from build123d import *

# Parameters (mm, degrees)
SKETCH_1_R          = 18
SKETCH_1_R_2        = 1.55
EXTRUDE_1_DEPTH     = 4
SKETCH_3_R          = 2.6
CUT_EXTRUDE_2_DEPTH = 2
CUT_EXTRUDE_3_DEPTH = 26.53429067
SKETCH_5_R          = 5.1
EXTRUDE_2_DEPTH     = 6
CUT_EXTRUDE_START   = 2.4
SKETCH_2_R          = 1.55
CUT_EXTRUDE_4_DEPTH = 2.4


with BuildPart() as part:
    # Sketch 1 → Extrude 1 (new body)
    with BuildSketch(Plane(origin=(0, 0, 0), x_dir=(1, 0, 0), z_dir=(0, 1, 0))):
        with Locations(Location((0, 0, 0), (0, 0, 270))):
            Circle(SKETCH_1_R)
        with Locations(Location((-12.124355653, -7, 0), (0, 0, 270))):
            Circle(SKETCH_1_R_2, mode=Mode.SUBTRACT)
        with Locations(Location((0, 14, 0), (0, 0, 270))):
            Circle(SKETCH_1_R_2, mode=Mode.SUBTRACT)
        with Locations(Location((12.124355653, -7, 0), (0, 0, 270))):
            Circle(SKETCH_1_R_2, mode=Mode.SUBTRACT)
    extrude(amount=EXTRUDE_1_DEPTH)

    # Sketch 3 → Cut-Extrude 2 (cut)
    with BuildSketch(Plane.XZ):
        with Locations(Location((0, 0, 0), (0, 0, 270))):
            Circle(SKETCH_3_R)
    extrude(amount=-CUT_EXTRUDE_2_DEPTH, mode=Mode.SUBTRACT)

    # Sketch 4 → Cut-Extrude 3 (cut, through all)
    with BuildSketch(Plane.XZ.offset(-2)):
        with BuildLine():
            ThreePointArc((2.6, 0), (-1.177768117, 2.317943542), (-1.532970972, -2.1))
            Line((-1.532970972, -2.1), (1.532970972, -2.1))
            ThreePointArc((1.532970972, -2.1), (2.317943542, -1.177768117), (2.6, 0))
        make_face()
    extrude(amount=-CUT_EXTRUDE_3_DEPTH, mode=Mode.SUBTRACT)

    # Sketch 5 → Extrude 2 (add)
    with BuildSketch(Plane(origin=(0, 4, 0), x_dir=(1, 0, 0), z_dir=(0, 1, 0))):
        with Locations(Location((0, 0, 0), (0, 0, 270))):
            Circle(SKETCH_5_R)
        with BuildLine():
            Line((-1.532970972, 2.1), (1.532970972, 2.1))
            ThreePointArc((1.532970972, 2.1), (0, -2.6), (-1.532970972, 2.1))
        make_face(mode=Mode.SUBTRACT)
    extrude(amount=EXTRUDE_2_DEPTH)

    # Sketch 2 → Cut-Extrude 4 (cut)
    # profile 1 of 3: a face of its own
    with BuildSketch(Plane.XZ.offset(-4).offset(CUT_EXTRUDE_START)):
        Polygon((-8.891194146, 7), (-10.507774899, 9.8), (-13.740936407, 9.8), (-15.35751716, 7), (-13.740936407, 4.2), (-10.507774899, 4.2), align=None)
        with Locations(Location((-12.124355653, 7, 0), (0, 0, 270))):
            Circle(SKETCH_2_R, mode=Mode.SUBTRACT)
    # profile 2 of 3: a face of its own
    with BuildSketch(Plane.XZ.offset(-4).offset(CUT_EXTRUDE_START)):
        Polygon((-1.616580754, -11.2), (-3.233161507, -14), (-1.616580754, -16.8), (1.616580754, -16.8), (3.233161507, -14), (1.616580754, -11.2), align=None)
        with Locations(Location((0, -14, 0), (0, 0, 270))):
            Circle(SKETCH_2_R, mode=Mode.SUBTRACT)
    # profile 3 of 3: a face of its own
    with BuildSketch(Plane.XZ.offset(-4).offset(CUT_EXTRUDE_START)):
        Polygon((10.507774899, 4.2), (13.740936407, 4.2), (15.35751716, 7), (13.740936407, 9.8), (10.507774899, 9.8), (8.891194146, 7), align=None)
        with Locations(Location((12.124355653, 7, 0), (0, 0, 270))):
            Circle(SKETCH_2_R, mode=Mode.SUBTRACT)
    extrude(amount=-CUT_EXTRUDE_4_DEPTH, mode=Mode.SUBTRACT)


solid = part.part
CAD build for the part. Positions are in the model's coordinates, mm. A direction names the side the tool comes from. Give positions to 0.01 mm unless a question says otherwise; leave off trailing zeros. Write each loop counter-clockwise with the first axis right and the second up, starting at its lowest first coordinate (ties: lowest second). Pieces come first, ordered by that corner, then holes. Notation, with made-up numbers: M -21,42.5 L 14,42.5 A22 ccw 14,62.5 Z; hole C 14.25,57 d6. An arc over 180 degrees is marked long. Put each result on its own line as item: value. Start each with the question number.
(1) Band-saw the part on A-A, the plane x = 0. Write the cut outline in (y, z), and give its area (3 significant figures).
(2) Band-saw the part on D-D, the plane z = 9. Write the cut outline in (x, y).
(3) Flat gauge pins, fed straight in: pin 1 Ø4 at (x, z) = (0, 0) entering from -Y; pin 2 Ø3 at (x, z) = (-0.5, -13) entering from +Y; pin 3 Ø1.9 at (x, y) = (-12.5, 3) entering from -Z; pin 4 Ø6 at (x, z) = (-7, -13) entering from +Y. Where does each tip first touch, or does it go through?
(4) Band-saw the part on C-C, the plane x = 11. Write the cut outline in (y, z).
(5) Band-saw the part on B-B, the plane y = 3.5. Write the cut outline in (x, z), and give its area (3 significant figures).
(6) Probe L1, parallel to Z at x = 1, y = 3.5; L2, parallel to X at y = 3.5, z = 0; L3, parallel to X at y = 1.2, z = 7. List the from-to ranges inside material, lowest first.
(7) Mould opens along X. For faces 4 (the face through (-14.538, 2.783, 8.42)), 5 (the face through (14.538, 2.783, 5.58)), 6 (the face through (-4, 4, 4)) say: +X half, -X half, draft (parallel to the pull), parting line (faces both ways), or undercut.
(8) Which spindle directions (+Z, -Z, +X, -X, +Y, -Y) get a long thin tool onto all of the face, cutting with end or side? Do faces 1 (the face through (0, 6, -2.1)), 2 (the face through (-12, 3, 4.2)), 3 (the face through (-4, 0, 0)). Say none if no direction does.
Response values:
1. outline: M 0,-18 L 4,-18 L 4,-16.8 L 1.6,-16.8 L 1.6,-15.55 L 0,-15.55 Z; M 0,-12.45 L 1.6,-12.45 L 1.6,-11.2 L 4,-11.2 L 4,-5.1 L 10,-5.1 L 10,-2.1 L 2,-2.1 L 2,-2.6 L 0,-2.6 Z; M 0,2.6 L 10,2.6 L 10,5.1 L 4,5.1 L 4,18 L 0,18 Z
1. area: 139 mm2
2. outline: M -15.59,0 L 15.59,0 L 15.59,4 L 14.2,4 L 14.2,1.6 L 10.05,1.6 L 10.05,4 L -10.05,4 L -10.05,1.6 L -14.2,1.6 L -14.2,4 L -15.59,4 Z
3. pin 1: passes through
3. pin 2: stops at y = 1.6
3. pin 3: stops at z = -13.81
3. pin 4: stops at y = 4
4. outline: M 0,-14.25 L 4,-14.25 L 4,4.2 L 1.6,4.2 L 1.6,5.93 L 0,5.93 Z; M 0,8.07 L 1.6,8.07 L 1.6,9.8 L 4,9.8 L 4,14.25 L 0,14.25 Z
5. outline: C 0,0 d36; hole M -15.36,7 L -13.74,4.2 L -10.51,4.2 L -8.89,7 L -10.51,9.8 L -13.74,9.8 Z; hole M -3.23,-14 L -1.62,-16.8 L 1.62,-16.8 L 3.23,-14 L 1.62,-11.2 L -1.62,-11.2 Z; hole M -1.53,-2.1 L 1.53,-2.1 A2.6 ccw long Z; hole M 8.89,7 L 10.51,4.2 L 13.74,4.2 L 15.36,7 L 13.74,9.8 L 10.51,9.8 Z
5. area: 916 mm2
6. L1: z = -17.97 to -16.8, -11.2 to -2.1, 2.4 to 17.97
6. L2: x = -18 to -2.6, 2.6 to 18
6. L3: x = -16.58 to -13.67, -10.57 to 10.57, 13.67 to 16.58
7. face 4: undercut
7. face 5: undercut
7. face 6: draft
8. face 1: +Y, -Y
8. face 2: +Y
8. face 3: +Z, -Z, +X, -X, -Y
